Read the model definition and answer for the solid it produces. Units are mm, in the model's axes. Face numbers are marked on the shaded views. A direction names the side the tool comes from. Give positions to 0.01 mm unless a question says otherwise; leave off trailing zeros. Write each loop counter-clockwise with the first axis right and the second up, starting at its lowest first coordinate (ties: lowest second). Pieces come first, ordered by that corner, then holes. Notation, with made-up numbers: (23.25, 82.5) - (30.25, 82.5) arc R27 ccw to (30.25, 100.5) - close; hole circle Ø2 at (-12.5, -30). An arc over 180 degrees is marked (long way). Answer as CSV lines item,"result".
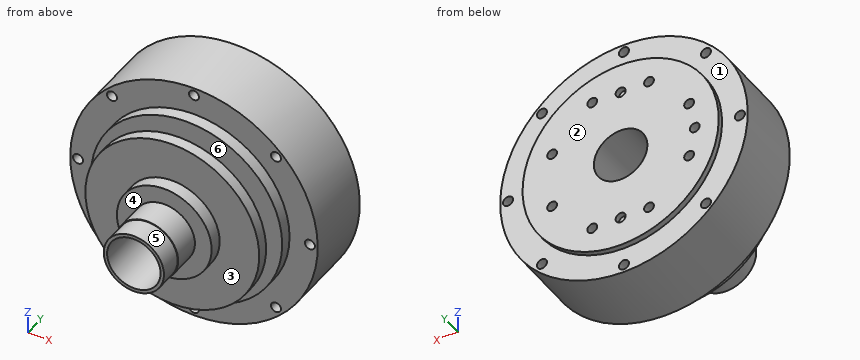
```python
from build123d import *

# Parameters (mm, degrees)
SKETCH2_R          = 4.5
CUT_EXTRUDE1_DEPTH = 220.205383146
SKETCH4_R          = 4.4
CUT_EXTRUDE3_DEPTH = 18
SKETCH5_R          = 4.5
CUT_EXTRUDE4_DEPTH = 5
SKETCH6_R          = 24
CUT_EXTRUDE5_DEPTH = 223.724044504


with BuildPart() as part:
    # Sketch1 → Revolve1 (revolve)
    with BuildSketch(Plane(origin=(0, 0, 0), x_dir=(0, 0, -1), z_dir=(1, 0, 0)), mode=Mode.PRIVATE) as revolve1_sk:
        Polygon((0, 0), (-27, 0), (-27, 20.5), (-27.5, 20.5), (-27.5, 45.55), (-42.5, 45.55), (-42.5, 57.55), (-78, 57.55), (-78, 67.843005088), (-42.911855869, 67.843005088), (-42.911855869, 74.568826386), (-50.146203661, 74.568826386), (-50.146203661, 79), (-85.75, 79), (-85.75, 90), (-111, 90), (-111, 153), (-88, 153), (-88, 158), (0, 158), align=None)
    revolve(revolve1_sk.sketch.rotate(Axis((0, 0, 0), (0, 1, 0)), 180), axis=Axis((0, 0, 0), (0, 1, 0)))

    # Sketch2 → Cut-Extrude1 (cut, through all)
    with BuildSketch(Plane(origin=(0, 153, 0), x_dir=(1, 0, 0), z_dir=(0, 1, 0))):
        with Locations(Location((-104, 0, 0), (0, 0, 270))):
            Circle(SKETCH2_R)
        with Locations(Location((-73.539105243, 73.539105243, 0), (0, 0, 270))):
            Circle(SKETCH2_R)
        with Locations(Location((0, 104, 0), (0, 0, 270))):
            Circle(SKETCH2_R)
        with Locations(Location((73.539105243, 73.539105243, 0), (0, 0, 270))):
            Circle(SKETCH2_R)
        with Locations(Location((104, 0, 0), (0, 0, 270))):
            Circle(SKETCH2_R)
        with Locations(Location((73.539105243, -73.539105243, 0), (0, 0, 270))):
            Circle(SKETCH2_R)
        with Locations(Location((0, -104, 0), (0, 0, 270))):
            Circle(SKETCH2_R)
        with Locations(Location((-73.539105243, -73.539105243, 0), (0, 0, 270))):
            Circle(SKETCH2_R)
    extrude(amount=-CUT_EXTRUDE1_DEPTH, mode=Mode.SUBTRACT)

    # Sketch4 → Cut-Extrude3 (cut)
    with BuildSketch(Plane(origin=(0, 158, 0), x_dir=(1, 0, 0), z_dir=(0, 1, 0))):
        with Locations(Location((-66.5, 0, 0), (0, 0, 270))):
            Circle(SKETCH4_R)
        with Locations(Location((-61.437988912, 25.448448252, 0), (0, 0, 270))):
            Circle(SKETCH4_R)
        with Locations(Location((-25.448448252, 61.437988912, 0), (0, 0, 270))):
            Circle(SKETCH4_R)
        with Locations(Location((25.448448252, 61.437988912, 0), (0, 0, 270))):
            Circle(SKETCH4_R)
        with Locations(Location((61.437988912, 25.448448252, 0), (0, 0, 270))):
            Circle(SKETCH4_R)
        with Locations(Location((61.437988912, -25.448448252, 0), (0, 0, 270))):
            Circle(SKETCH4_R)
        with Locations(Location((25.448448252, -61.437988912, 0), (0, 0, 270))):
            Circle(SKETCH4_R)
        with Locations(Location((-25.448448252, -61.437988912, 0), (0, 0, 270))):
            Circle(SKETCH4_R)
        with Locations(Location((-61.437988912, -25.448448252, 0), (0, 0, 270))):
            Circle(SKETCH4_R)
    extrude(amount=-CUT_EXTRUDE3_DEPTH, mode=Mode.SUBTRACT)

    # Sketch5 → Cut-Extrude4 (cut)
    with BuildSketch(Plane(origin=(0, 158, 0), x_dir=(1, 0, 0), z_dir=(0, 1, 0))):
        with Locations(Location((0, -61.25, 0), (0, 0, 270))):
            Circle(SKETCH5_R)
        with Locations(Location((0, 61.25, 0), (0, 0, 270))):
            Circle(SKETCH5_R)
    extrude(amount=-CUT_EXTRUDE4_DEPTH, mode=Mode.SUBTRACT)

    # Sketch6 → Cut-Extrude5 (cut, through all)
    with BuildSketch(Plane.XZ):
        with Locations(Location((0, 0, 0), (0, 0, 270))):
            Circle(SKETCH6_R)
    extrude(amount=-CUT_EXTRUDE5_DEPTH, mode=Mode.SUBTRACT)


solid = part.part
```
(1) Each of these flat-tipped pins is pushed along its axis until it touches: P1, Ø8, axis at x = 38.5, y = 115, coming from the +Z side; P2, Ø6, axis at x = 74.5, z = -58, coming from the -Y side; P3, Ø8, axis at x = 0, z = 61.25, coming from the +Y side. Where does it stop, or does it pass through?
Worked out:
P1,"stops at z = 105.5"
P2,"stops at y = 90"
P3,"stops at y = 153"
(2) A cutting plane is placed at B-B (x = 104). Write down the section's boundary in (y, z).
Worked out:
outline,"(90, -38.79) - (153, -38.79) - (153, -4.5) - (90, -4.5) - close; (90, 4.5) - (153, 4.5) - (153, 38.79) - (90, 38.79) - close"
(3) A cutting plane is placed at A-A (y = 146). Count the separate pieces of the cut face and the enclosed holes in it, and give its area (3 significant figures).
Worked out:
separate pieces,"1"
enclosed holes,"18"
area,"35,800 mm^2"
(4) The mould has two halves that part along Y. Classify the marked faces 4, 5 and 6: +Y half, -Y half, draft (parallel to the pull), parting line (faces both ways), or undercut.
Worked out:
face 4,"-Y half"
face 5,"draft"
face 6,"undercut"
(5) Find the intervals of material crossed by L1, parallel to Y at x = 31.5, z = 59; L2, parallel to Z at x = -73, y = 143.5; L3, parallel to Y at x = -14, z = 28, in increasing order.
Worked out:
L1,"y = 57.55 to 67.84, 79 to 158"
L2,"z = -83.62 to -78.01, -69.07 to 69.07, 78.01 to 83.62"
L3,"y = 45.55 to 158"
(6) For the marked faces 1, 2 and 3, determine the directions among +Z, -Z, +X, -X, +Y, -Y from which every point of the face is accessible in a straight line to the end or side of a thin tool.
Worked out:
face 1,"+Y"
face 2,"+Z, -Z, +X, -X, +Y"
face 3,"-Y"
(7) A cutting plane is placed at C-C (z = -61.25). Write down the section's boundary in (x, y), and give its area (3 significant figures).
Worked out:
outline,"(-92.57, 90) - (-60.01, 90) - (-60.01, 79) - (60.01, 79) - (60.01, 90) - (92.57, 90) - (92.57, 153) - (63.19, 153) - (63.19, 158) - (29.84, 158) - (29.84, 140) - (21.05, 140) - (21.05, 158) - (4.5, 158) - (4.5, 153) - (-4.5, 153) - (-4.5, 158) - (-21.05, 158) - (-21.05, 140) - (-29.84, 140) - (-29.84, 158) - (-63.19, 158) - (-63.19, 153) - (-92.57, 153) - close; (-48.3, 57.55) - (48.3, 57.55) - (48.3, 67.84) - (-48.3, 67.84) - close"
area,"14,200 mm^2"
